```python
from build123d import *

# Parameters (mm, degrees)
SKETCH1_R           = 22.5
BOSS_EXTRUDE1_DEPTH = 141.739806
SKETCH2_R           = 17.803613723
CUT_EXTRUDE1_DEPTH  = 146.267589658


with BuildPart() as part:
    # Sketch1 → Boss-Extrude1 (new body)
    with BuildSketch(Plane(origin=(0, 0, 0), x_dir=(1, 0, 0), z_dir=(0, 1, 0))):
        with Locations(Location((0, 0, 0), (0, 0, 270))):
            Circle(SKETCH1_R)
    extrude(amount=BOSS_EXTRUDE1_DEPTH)

    # Sketch2 → Cut-Extrude1 (cut, through all)
    with BuildSketch(Plane(origin=(0, 0, 0), x_dir=(1, 0, 0), z_dir=(0, 1, 0))):
        with Locations(Location((0, 0, 0), (0, 0, 270))):
            Circle(SKETCH2_R)
    extrude(amount=CUT_EXTRUDE1_DEPTH, mode=Mode.SUBTRACT)

    # Chamfer1: read off the stored shape, not the designer's step
    # Chamfer1 outline → Chamfer1 (revolve, cut)
    with BuildSketch(Plane.XY):
        Polygon((22.5, 136.88216168), (22.5, 141.73980616), (17.803613723, 141.73980616), (17.803613723, 141.578547956), align=None)
        Polygon((22.5, 4.857644481), (17.803613723, 0.161258204), (17.803613723, 0), (22.5, 0), align=None)
    revolve(axis=Axis((0, 0, 0), (0, 1, 0)), mode=Mode.SUBTRACT)


solid = part.part
```
Model file for the job. Use its own axes, mm. Coordinates: 2 decimals unless noted, no trailing zeros. Loops run counter-clockwise (first coordinate to the right, second up) from the corner with the lowest first, then second, coordinate; pieces in that order, holes last. Notation, with made-up numbers: M 39.25,-5.75 L 85.25,-5.75 A27 ccw 85.25,12.25 Z; hole C -9.75,43.25 d4. An arc over 180 degrees is marked long. Use CSV: the item, a comma, the result in double quotes. Start each with the question number.
1. Probe probe 1 along Z at (x, y) = (0, 47); probe 2 along X at (y, z) = (19.5, -13.5). List the from-to ranges inside material, lowest first. Write a range as [from, to].
2. Two-plate mould, pull along Z, no slides. Class faces 1 (the cylindrical face through (5.35, 69.88, 16.98)), 2 (the conical face through (-14.3, 0.4, 11)): pulls with the +Z half, pulls with the -Z half, needs draft (parallel to the pull), parting line crosses it, or undercut.
3. Flat gauge pins, fed straight in: pin 1 (1 mm diameter, centred on y = 109.5, z = 7, fed in from -X); pin 2 (8 mm diameter, centred on x = -5, y = 106.5, fed in from -Z); pin 3 (2 mm diameter, centred on y = 63.5, z = 16, fed in from +X); pin 4 (12 mm diameter, centred on x = -0.5, z = -6.5, fed in from +Y). Where does each tip first touch, or does it go through?
4. Band-saw the part on B-B, the plane x = 0. List the corners of the cut face in (y, z), then the cut area to 3 significant figures.
5. Band-saw the part on C-C, the plane y = 39. List the corners of the cut face in (x, z), then the cut area to 3 significant figures.
6. Band-saw the part on A-A, the plane z = 0. List the corners of the cut face in (x, y), then the cut area to 3 significant figures.
Entries:
1,probe 1,"z = [-22.5, -17.8], [17.8, 22.5]"
1,probe 2,"x = [-18, -11.61], [11.61, 18]"
2,face 1,"undercut"
2,face 2,"parting line crosses it"
3,pin 1,"stops at x = -21.54"
3,pin 2,"stops at z = -22.48"
3,pin 3,"stops at x = 16.77"
3,pin 4,"passes through"
4,outline,"M 0.16,-17.8 L 4.86,-22.5 L 136.88,-22.5 L 141.58,-17.8 Z; M 0.16,17.8 L 141.58,17.8 L 136.88,22.5 L 4.86,22.5 Z"
4,area,"1,280 mm2"
5,outline,"C 0,0 d45; hole C 0,0 d35.61"
5,area,"595 mm2"
6,outline,"M -22.5,4.86 L -17.8,0.16 L -17.8,141.58 L -22.5,136.88 Z; M 17.8,0.16 L 22.5,4.86 L 22.5,136.88 L 17.8,141.58 Z"
6,area,"1,280 mm2"
